The listing builds one solid part. Answer for the finished solid, in the listing's coordinates (mm). A direction names the side the tool comes from. Coordinates: 2 decimals unless noted, no trailing zeros. Order: outer loops, then holes, each group sorted by start corner. A loop starts at its lowest first (then second) coordinate and runs counter-clockwise, first axis right, second up. Notation, with made-up numbers: (55.25, 55) -> (99.25, 55) arc R6 ccw to (99.25, 64) -> close; hole circle Ø5 at (77.25, 19.5). An arc over 180 degrees is marked (long way). Return JSON: item names as keys, results as strings.
```python
from build123d import *

# Parameters (mm, degrees)
F1_DEPTH = 5
F3_DEPTH = 4
F4_R     = 2
F5_R     = 1.25
F6_DEPTH = 5.001


with BuildPart() as f1:
    # F0 (on Top) → F1 (new body)
    with BuildSketch(Plane.XY):
        with BuildLine():
            Line((-18, -21.5), (18, -21.5))
            ThreePointArc((18, -21.5), (21.535534, -20.035534), (23, -16.5))
            Line((23, -16.5), (23, 16.5))
            ThreePointArc((23, 16.5), (21.535534, 20.035534), (18, 21.5))
            Line((18, 21.5), (-18, 21.5))
            ThreePointArc((-18, 21.5), (-21.535534, 20.035534), (-23, 16.5))
            Line((-23, 16.5), (-23, -16.5))
            ThreePointArc((-23, -16.5), (-21.535534, -20.035534), (-18, -21.5))
        make_face()
    extrude(amount=F1_DEPTH)

    # F2 (on face) → F3 (cut)
    with BuildSketch(Plane.XY.offset(5)):
        with BuildLine():
            Line((-18, -20), (18, -20))
            ThreePointArc((18, -20), (20.474874, -18.974874), (21.5, -16.5))
            Line((21.5, -16.5), (21.5, 16.5))
            ThreePointArc((21.5, 16.5), (20.474874, 18.974874), (18, 20))
            Line((18, 20), (-18, 20))
            ThreePointArc((-18, 20), (-20.474874, 18.974874), (-21.5, 16.5))
            Line((-21.5, 16.5), (-21.5, -16.5))
            ThreePointArc((-21.5, -16.5), (-20.474874, -18.974874), (-18, -20))
        make_face()
    extrude(amount=-F3_DEPTH, mode=Mode.SUBTRACT)

    # F4
    f4_edges = [f1.edges().sort_by_distance(p)[0] for p in [
        (-21.535534, -20.035534, 0),
        (0, -21.5, 0),
        (21.535534, -20.035534, 0),
        (23, 0, 0),
        (21.535534, 20.035534, 0),
        (0, 21.5, 0),
        (-21.535534, 20.035534, 0),
        (-23, 0, 0),
    ]]
    fillet(f4_edges, radius=F4_R)

    # F5 (on face) → F6 (cut, through all)
    with BuildSketch(Plane(origin=(0, 0, 0), x_dir=(1, 0, 0), z_dir=(0, 0, -1))):
        with Locations((-18, 16.5)):
            Circle(F5_R)
        with Locations((18, 16.5)):
            Circle(F5_R)
        with Locations((18, -16.5)):
            Circle(F5_R)
        with Locations((-18, -16.5)):
            Circle(F5_R)
    extrude(amount=-F6_DEPTH, mode=Mode.SUBTRACT)


solid = f1.part
```
Item 1: Flat-ended cylindrical pins translate along their axes: pin 1 (3 mm diameter, centred on x = 14, y = -12, fed in from +Z); pin 2 (2 mm diameter, centred on x = 18, y = -16.5, fed in from +Z). Find the tip coordinate at first contact, or state that the pin passes through.
Answer list:
{"pin 1": "z = 1", "pin 2": "through"}
Item 2: The part is cut by section B-B on x = 9. Determine the outline of the cut face in (y, z), plus the area to 3 significant figures.
Answer list:
{"outline": "(-21.5, 2) arc R2 ccw to (-19.5, 0) -> (19.5, 0) arc R2 ccw to (21.5, 2) -> (21.5, 5) -> (20, 5) -> (20, 1) -> (-20, 1) -> (-20, 5) -> (-21.5, 5) -> close", "area": "53.3 mm2"}
Item 3: The part is cut by section C-C on y = -5. Determine the outline of the cut face in (x, z), plus the area to 3 significant figures.
Answer list:
{"outline": "(-23, 2) arc R2 ccw to (-21, 0) -> (21, 0) arc R2 ccw to (23, 2) -> (23, 5) -> (21.5, 5) -> (21.5, 1) -> (-21.5, 1) -> (-21.5, 5) -> (-23, 5) -> close", "area": "56.3 mm2"}
Item 4: The part is cut by section A-A on z = 3.05. Determine the outline of the cut face in (x, y), plus the area to 3 significant figures.
Answer list:
{"outline": "(-23, -16.5) arc R5 ccw to (-18, -21.5) -> (18, -21.5) arc R5 ccw to (23, -16.5) -> (23, 16.5) arc R5 ccw to (18, 21.5) -> (-18, 21.5) arc R5 ccw to (-23, 16.5) -> close; hole (-21.5, -16.5) arc R3.5 ccw to (-18, -20) -> (18, -20) arc R3.5 ccw to (21.5, -16.5) -> (21.5, 16.5) arc R3.5 ccw to (18, 20) -> (-18, 20) arc R3.5 ccw to (-21.5, 16.5) -> close", "area": "247 mm2"}
Item 5: Find the intervals of material crossed by probe 1 along Y at (x, z) = (14, 3.5); probe 2 along X at (y, z) = (10, 3.45); probe 3 along X at (y, z) = (-16.5, 0.65), in increasing order.
Answer list:
{"probe 1": "-21.5 to -20, 20 to 21.5", "probe 2": "-23 to -21.5, 21.5 to 23", "probe 3": "-22.48 to -19.25, -16.75 to 16.75, 19.25 to 22.48"}
Item 6: Which of the six approach directions +Z, -Z, +X, -X, +Y, -Y give full straight-line access (tool end or side, diameter ignored) to faces 4 (the flat face through (0, -21.5, 3)), 5 (the cylindrical face through (20.45, -19, 3.03))?
Answer list:
{"face 4": "+Z, -Z, +X, -X, -Y", "face 5": "+Z"}
Item 7: Determine the mould class of faces 1 (the cylindrical face through (-21.5, 20.07, 3.48)), 2 (the cylindrical face through (18.672, -17.554, 0.493)), 3 (the flat face through (0, -21, 5)) for opening direction X: pulls with the +X half, pulls with the -X half, needs draft (parallel to the pull), parting line crosses it, or undercut.
Answer list:
{"face 1": "pulls with the -X half", "face 2": "undercut", "face 3": "needs draft"}
